```python
from build123d import *

# Parameters (mm, degrees)
SKETCH1_W           = 101.6
SKETCH1_H           = 76.2
BOSS_EXTRUDE1_DEPTH = 3
SKETCH2_W           = 50.8
SKETCH2_H           = 3
CUT_EXTRUDE1_DEPTH  = 3
CUT_EXTRUDE2_DEPTH  = 3


with BuildPart() as part:
    # Sketch1 → Boss-Extrude1 (new body)
    with BuildSketch(Plane(origin=(0, 0, 0), x_dir=(1, 0, 0), z_dir=(0, 1, 0))):
        with Locations((50.8, 38.1)):
            Rectangle(SKETCH1_W, SKETCH1_H)
    extrude(amount=BOSS_EXTRUDE1_DEPTH)

    # Sketch2 → Cut-Extrude1 (cut)
    with BuildSketch(Plane(origin=(0, 3, 0), x_dir=(1, 0, 0), z_dir=(0, 1, 0))):
        with Locations((76.2, 25.4)):
            Rectangle(SKETCH2_W, SKETCH2_H)
    extrude(amount=-CUT_EXTRUDE1_DEPTH, mode=Mode.SUBTRACT)

    # Sketch3 → Cut-Extrude2 (cut)
    with BuildSketch(Plane(origin=(0, 3, 0), x_dir=(1, 0, 0), z_dir=(0, 1, 0))):
        Polygon((15, 51.2), (23.660254038, 56.2), (23.660254038, 66.2), (15, 71.2), (6.339745962, 66.2), (6.339745962, 56.2), align=None)
    extrude(amount=-CUT_EXTRUDE2_DEPTH, mode=Mode.SUBTRACT)


solid = part.part
```
CAD build for the part. Positions are in the model's coordinates, mm. A direction names the side the tool comes from. Round coordinates to 2 decimals unless told otherwise and drop trailing zeros. Order: outer loops, then holes, each group sorted by start corner. A loop starts at its lowest first (then second) coordinate and runs counter-clockwise, first axis right, second up.
Item 1: Probe line 1 along Z through (x, y) = (51, 1.15); line 2 along X through (y, z) = (2.6, -58); line 3 along X through (y, z) = (1.45, -52.5). List the from-to ranges inside material, lowest first.
Item 2: Tool access for faces 4 (the face through (19.27, 1.521, -53.665)), 5 (the face through (50.8, 2, -25)), 6 (the face through (0, 1, -38)): list every direction of +Z, -Z, +X, -X, +Y, -Y with a clear straight run to the whole face (end or side of a thin tool).
Item 3: Mould opens along Z. For faces 1 (the face through (50, 1, -76.2)), 2 (the face through (10.73, 1.521, -68.735)), 3 (the face through (101.6, 1, -51)) say: pulls with the +Z half, pulls with the -Z half, needs draft (parallel to the pull), parting line crosses it, or undercut.
Item 4: Pin check, flat tip, straight feed: pin 1 (1.5 mm diameter, centred on x = 67.5, y = 1.5, fed in from +Z). Stop position of the tip, or through.
Item 5: Saw through at C-C on z = -55. Write the cut outline in (x, y), then the cut area to 3 significant figures.
Item 6: Saw through at A-A on x = 93. Write the cut outline in (y, z), then the cut area to 3 significant figures.
Item 7: Saw through at B-B on y = 1.9. Write the cut outline in (x, z).
Reported:
1. line 1: z = -76.2 to -26.9, -23.9 to 0
1. line 2: x = 0 to 6.34, 23.66 to 101.6
1. line 3: x = 0 to 12.75, 17.25 to 101.6
2. face 4: +Y, -Y
2. face 5: +X, +Y, -Y
2. face 6: +Z, -Z, -X, +Y, -Y
3. face 1: pulls with the -Z half
3. face 2: undercut
3. face 3: needs draft
4. pin 1: stops at z = 0
5. outline: (0, 0) - (8.42, 0) - (8.42, 3) - (0, 3) - close; (21.58, 0) - (101.6, 0) - (101.6, 3) - (21.58, 3) - close
5. area: 265 mm2
6. outline: (0, -76.2) - (3, -76.2) - (3, -26.9) - (0, -26.9) - close; (0, -23.9) - (3, -23.9) - (3, 0) - (0, 0) - close
6. area: 220 mm2
7. outline: (0, -76.2) - (101.6, -76.2) - (101.6, -26.9) - (50.8, -26.9) - (50.8, -23.9) - (101.6, -23.9) - (101.6, 0) - (0, 0) - close; hole (6.34, -66.2) - (15, -71.2) - (23.66, -66.2) - (23.66, -56.2) - (15, -51.2) - (6.34, -56.2) - close
